from build123d import *

# Parameters (mm, degrees)
BOSS_EXTRUDE1_START = 12.7
SKETCH3_R           = 11.1125
SKETCH3_R_2         = 6.3627
BOSS_EXTRUDE1_DEPTH = 3.175
BOSS_EXTRUDE2_START = 9.525
SKETCH4_R           = 7.9629
SKETCH4_R_2         = 6.3627
BOSS_EXTRUDE2_DEPTH = 22.225
CHAMFER1_SIZE       = 0.190881


with BuildPart() as part:
    # Sketch3 → Boss-Extrude1 (new body)
    with BuildSketch(Plane.XY.offset(BOSS_EXTRUDE1_START)):
        Circle(SKETCH3_R)
        Circle(SKETCH3_R_2, mode=Mode.SUBTRACT)
    extrude(amount=-BOSS_EXTRUDE1_DEPTH)

    # Sketch4 → Boss-Extrude2 (add)
    with BuildSketch(Plane.XY.offset(BOSS_EXTRUDE2_START)):
        Circle(SKETCH4_R)
        Circle(SKETCH4_R_2, mode=Mode.SUBTRACT)
    extrude(amount=-BOSS_EXTRUDE2_DEPTH)

    # Chamfer1
    chamfer1_edges = [part.edges().sort_by_distance(p)[0] for p in [
        (-6.3627, 0, -12.7),
        (-7.9629, 0, 9.525),
        (-11.1125, 0, 12.7),
        (-11.1125, 0, 9.525),
        (-6.3627, 0, 12.7),
        (-7.9629, 0, -12.7),
    ]]
    chamfer(chamfer1_edges, length=CHAMFER1_SIZE)


solid = part.part
The listing builds one solid part. Answer for the finished solid, in the listing's coordinates (mm). A direction names the side the tool comes from. Round coordinates to 2 decimals unless told otherwise and drop trailing zeros. Order: outer loops, then holes, each group sorted by start corner. A loop starts at its lowest first (then second) coordinate and runs counter-clockwise, first axis right, second up. Notation, with made-up numbers: (55, -25.5) -> (91, -25.5) arc R26 ccw to (91, -0.5) -> close; hole circle Ø10 at (24.5, 77.25). An arc over 180 degrees is marked (long way). Put each result on its own line as item: value.
Q1. Consider line 1 along Z through (x, y) = (7, 6.5) (3 decimals); line 2 along Y through (x, z) = (0, 2.75); line 3 along X through (y, z) = (2.5, -8.5). Determine where each line is inside the solid, lowest interval first.
Results list:
line 1: 9.525 to 12.7
line 2: -7.96 to -6.36, 6.36 to 7.96
line 3: -7.56 to -5.85, 5.85 to 7.56
Q2. Which of the six approach directions +Z, -Z, +X, -X, +Y, -Y give full straight-line access (tool end or side, diameter ignored) to faces 4 (the flat face through (-3, -6, -12.7)), 5 (the flat face through (-4.1, -7.23, 9.525))?
Results list:
face 4: -Z, +X, -X, +Y, -Y
face 5: -Z
Q3. Determine the mould class of faces 1 (the cylindrical face through (-0.83, 6.31, 0.18)), 2 (the cylindrical face through (10.6, 3.34, 11.13)), 3 (the flat face through (5, -5, 12.7)) for opening direction Y: pulls with the +Y half, pulls with the -Y half, needs draft (parallel to the pull), parting line crosses it, or undercut.
Results list:
face 1: undercut
face 2: parting line crosses it
face 3: needs draft
Q4. Section C-C, the plane z = -11 is taken. Write down the section's boundary in (x, y), and give its area (3 significant figures).
Results list:
outline: circle Ø15.93 at (0, 0); hole circle Ø12.73 at (0, 0)
area: 72.0 mm^2
Q5. Each of these flat-tipped pins is pushed along its axis until it touches: P1, Ø8, axis at x = -3.5, z = -7, coming from the +Y side; P2, Ø8, axis at y = 4.5, z = -5.5, coming from the +X side; P3, Ø6, axis at x = 5, z = 5, coming from the +Y side; P4, Ø10, axis at x = 0, y = 0, coming from the +Z side. Where does it stop, or does it pass through?
Results list:
P1: y = 7.96
P2: x = 7.95
P3: y = 7.71
P4: through
